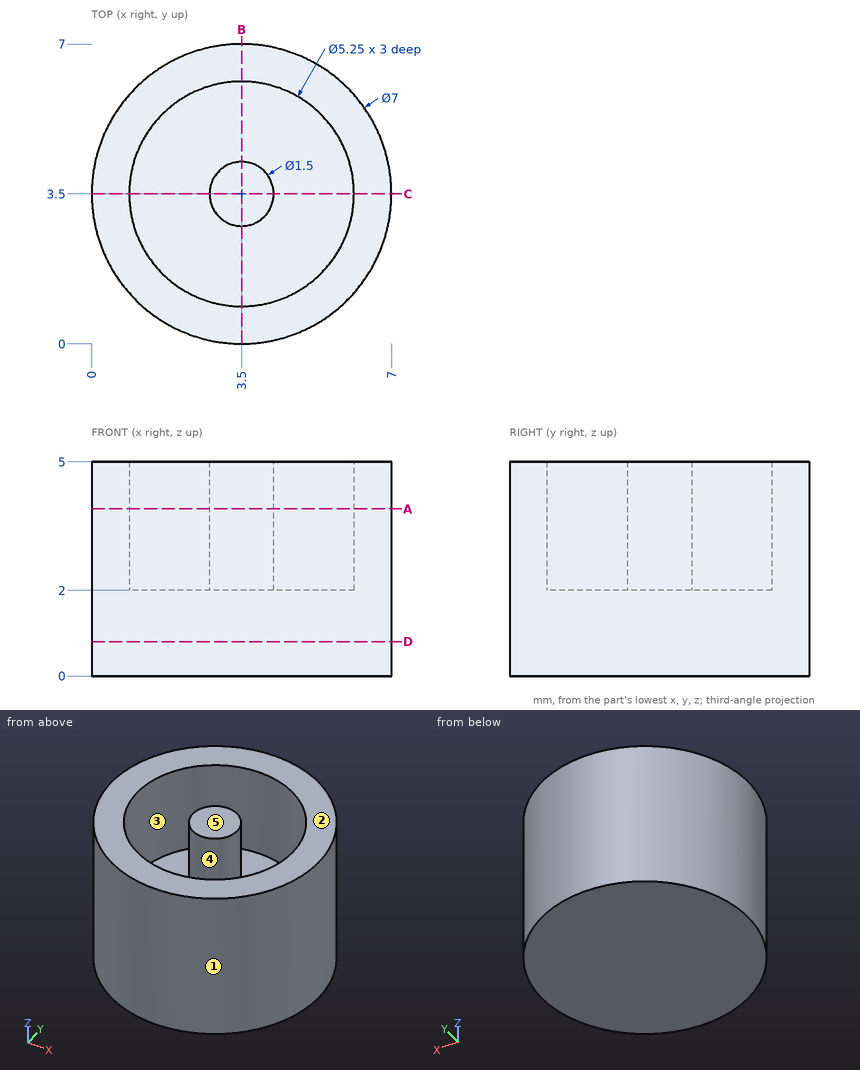
Check sheet for the drawn part. Datum: minimum x, y, z corner. Units: mm. A direction names the side the tool comes from. Give positions to 0.01 mm unless a question says otherwise; leave off trailing zeros. Write each loop counter-clockwise with the first axis right and the second up, starting at its lowest first coordinate (ties: lowest second). Pieces come first, ordered by that corner, then holes. Notation, with made-up numbers: (52.25, 66.5) -> (110.25, 66.5) arc R19 cw to (110.25, 100.5) -> close; hole circle Ø8 at (30, 41). An arc over 180 degrees is marked (long way). Use one line per item in the form item = value. Start each with the question number.
1. Section check B-B (x = 3.5). Record the cut outline in (y, z) (3 decimals).
2. Mould release check, pull along X, two halves, no side actions. Record for the marked faces 1, 2 and 3: pulls with the +X half, pulls with the -X half, needs draft (parallel to the pull), parting line crosses it, or undercut.
3. Section check A-A (z = 3.9). Record the cut outline in (x, y) (3 decimals), and give its area (3 significant figures).
4. Access from +Z, -Z, +X, -X, +Y, -Y to the whole of each face (thin tool, end or side, straight path). Record for the marked faces 4 and 5.
5. Section check D-D (z = 0.8). Record the cut outline in (x, y).
6. Go/stop test with flat-tipped pins: P1, Ø1, axis at x = 5.5, z = 0.5, coming from the -Y side; P2, Ø3, axis at y = 1.5, z = 1, coming from the -X side. Record where each tip stops, or that it passes through.
7. Thickness scan on line 1 along Y through (x, z) = (3.5, 4.1) (3 decimals); line 2 along X through (y, z) = (4, 2.1); line 3 along X through (y, z) = (1.25, 2.05). Record the ranges inside material, lowest first. Write a range as from..to.
Conclusion:
q1.outline = (0, 0) -> (7, 0) -> (7, 5) -> (6.125, 5) -> (6.125, 2) -> (4.25, 2) -> (4.25, 5) -> (2.75, 5) -> (2.75, 2) -> (0.875, 2) -> (0.875, 5) -> (0, 5) -> close
q2.face_1 = parting line crosses it
q2.face_2 = needs draft
q2.face_3 = undercut
q3.outline = circle Ø7 at (3.5, 3.5); circle Ø1.5 at (3.5, 3.5); hole circle Ø5.25 at (3.5, 3.5)
q3.area = 18.6 mm²
q4.face_4 = +Z
q4.face_5 = +Z, +X, -X, +Y, -Y
q5.outline = circle Ø7 at (3.5, 3.5)
q6.P1 = 0.34
q6.P2 = 0.04
q7.line_1 = 0..0.875, 2.75..4.25, 6.125..7
q7.line_2 = 0.04..0.92, 2.94..4.06, 6.08..6.96
q7.line_3 = 0.82..2.15, 4.85..6.18
